```python
from build123d import *

# Parameters (mm, degrees)
PAD_DEPTH           = 9.75
FILLET_R            = 2
POCKET_DEPTH        = 0.5
PAD001_DEPTH        = 17.499961
LINEARPATTERN_COUNT = 18
LINEARPATTERN_PITCH = 1.029412
FILLET001_R         = 1.5


with BuildPart() as part:
    # Sketch → Pad (new body, symmetric)
    with BuildSketch(Plane.YZ):
        with BuildLine():
            Line((0, 0), (21.5, 0))
            Line((21.5, 0), (21.5, -9.7))
            Line((21.5, -9.7), (22.3, -9.7))
            ThreePointArc((22.3, -11.5), (23.2, -10.6), (22.3, -9.7))
            Line((22.3, -11.5), (19.5, -11.5))
            Line((19.5, -11.5), (19.5, -4.5))
            Line((19.5, -4.5), (0, -4.5))
            Line((0, -4.5), (0, 0))
        make_face()
    extrude(amount=PAD_DEPTH, both=True)

    # Fillet
    fillet_edges = [part.edges().sort_by_distance(p)[0] for p in [
        (9.75, 0, -2.25),
        (-9.75, 0, -2.25),
    ]]
    fillet(fillet_edges, radius=FILLET_R)

    # Sketch001 (on Face1 of Fillet) → Pocket (cut)
    with BuildSketch(Plane(origin=(0, 0, 0), x_dir=(0, -1, 0), z_dir=(0, 0, 1))):
        with BuildLine():
            ThreePointArc((-1, 7.749997), (-1.292892, 8.457106), (-2, 8.75))
            Line((-19.25, 8.75), (-2, 8.75))
            Line((-19.25, 8.75), (-19.25, -8.749961))
            Line((-19.25, -8.749961), (-2, -8.749961))
            ThreePointArc((-2, -8.749961), (-1.292922, -8.45708), (-1.000039, -7.750003))
            Line((-1, 7.749997), (-1.000039, -7.750003))
        make_face()
    extrude(amount=-POCKET_DEPTH, mode=Mode.SUBTRACT)

    # Sketch002 (on Face11 of Pocket) → Pad001 (join)
    with BuildSketch(Plane.YZ.offset(-8.749961)):
        Polygon((18.220588, -0.05), (18.220588, -0.5), (19.25, -0.5), (19.25, -0.05), (18.735294, -0.4), align=None)
    pad001 = extrude(amount=PAD001_DEPTH)

    # LinearPattern: Pad001 ×18
    with Locations(*[(0, -i * LINEARPATTERN_PITCH, 0) for i in range(1, LINEARPATTERN_COUNT)]):
        add(pad001)

    # Fillet001
    fillet001_edges = [part.edges().sort_by_distance(p)[0] for p in [
        (0, 21.5, 0),
    ]]
    fillet(fillet001_edges, radius=FILLET001_R)


solid = part.part
```
Verification items for the finished model (mm, model axes). A direction names the side the tool comes from. Round coordinates to 2 decimals unless told otherwise and drop trailing zeros. Write each loop counter-clockwise with the first axis right and the second up, starting at its lowest first coordinate (ties: lowest second). Pieces come first, ordered by that corner, then holes. Notation, with made-up numbers: (31, 57.5) - (40, 57.5) arc R20 cw to (40, 90.5) - close; hole circle Ø5 at (-36.75, 77). An arc over 180 degrees is marked (long way). Answer as a JSON object with one key per item and string values. Group by question number.
Q1. Go/stop test with flat-tipped pins: pin 1 Ø1.5 at (x, z) = (-3, -8.5) entering from -Y; pin 2 Ø1.5 at (x, y) = (-1.5, 7.5) entering from +Z; pin 3 Ø0.6 at (x, y) = (-0.5, 22) entering from +Z. Record where each tip stops, or that it passes through.
Q2. Section check C-C, the plane z = -6.5. Enter the section's corners in (x, y).
Q3. Tool access check on faces 1 (the flat face through (0, 19.5, -8)), 2 (the cylindrical face through (0.1, 23.2, -10.6)), 3 (the flat face through (0, 21.5, -6)). Record the directions out of +Z, -Z, +X, -X, +Y, -Y that give a thin tool (end or side, any length) a straight path to the whole face; none if there is none.
Q4. Thickness scan on line 1 (Y direction, x = 0.5, z = -6); line 2 (Y direction, x = -4.5, z = -2.5); line 3 (Z direction, x = -3.5, y = 22). Record the ranges inside material, lowest first.
Q5. Section check A-A, the plane z = -2. Enter the section's corners in (x, y), plus the area to 3 significant figures.
Q6. Section check B-B, the plane z = -10.6. Enter the section's corners in (x, y).
Q7. Mould release check, pull along Y, two halves, no side actions. Record for faces 4 (the flat face through (-9, 9, 0)), 5 (the cylindrical face through (8.315, 1.175, -0.153)), 6 (the flat face through (0, 0, -2)), 7 (the cylindrical face through (-8.333, 1.187, -0.153)): released by +Y, released by -Y, zero draft, split by the parting line, or undercut.
Found:
{
 "1": {"pin 1": "stops at y = 19.5", "pin 2": "stops at z = -0.05", "pin 3": "stops at z = -9.7"},
 "2": {"outline": "(-9.75, 19.5) - (9.75, 19.5) - (9.75, 21.5) - (-9.75, 21.5) - close"},
 "3": {"face 1": "-Z, +X, -X, -Y", "face 2": "+X, -X, +Y", "face 3": "+Z, +X, -X, +Y"},
 "4": {"line 1": "y = 19.5 to 21.5", "line 2": "y = 0 to 21.5", "line 3": "z = -11.5 to -9.7"},
 "5": {"outline": "(-9.75, 2) arc R2 ccw to (-7.75, 0) - (7.75, 0) arc R2 ccw to (9.75, 2) - (9.75, 21.5) - (-9.75, 21.5) - close", "area": "418 mm^2"},
 "6": {"outline": "(-9.75, 19.5) - (9.75, 19.5) - (9.75, 23.2) - (-9.75, 23.2) - close"},
 "7": {"face 4": "zero draft", "face 5": "undercut", "face 6": "released by -Y", "face 7": "undercut"}
}
